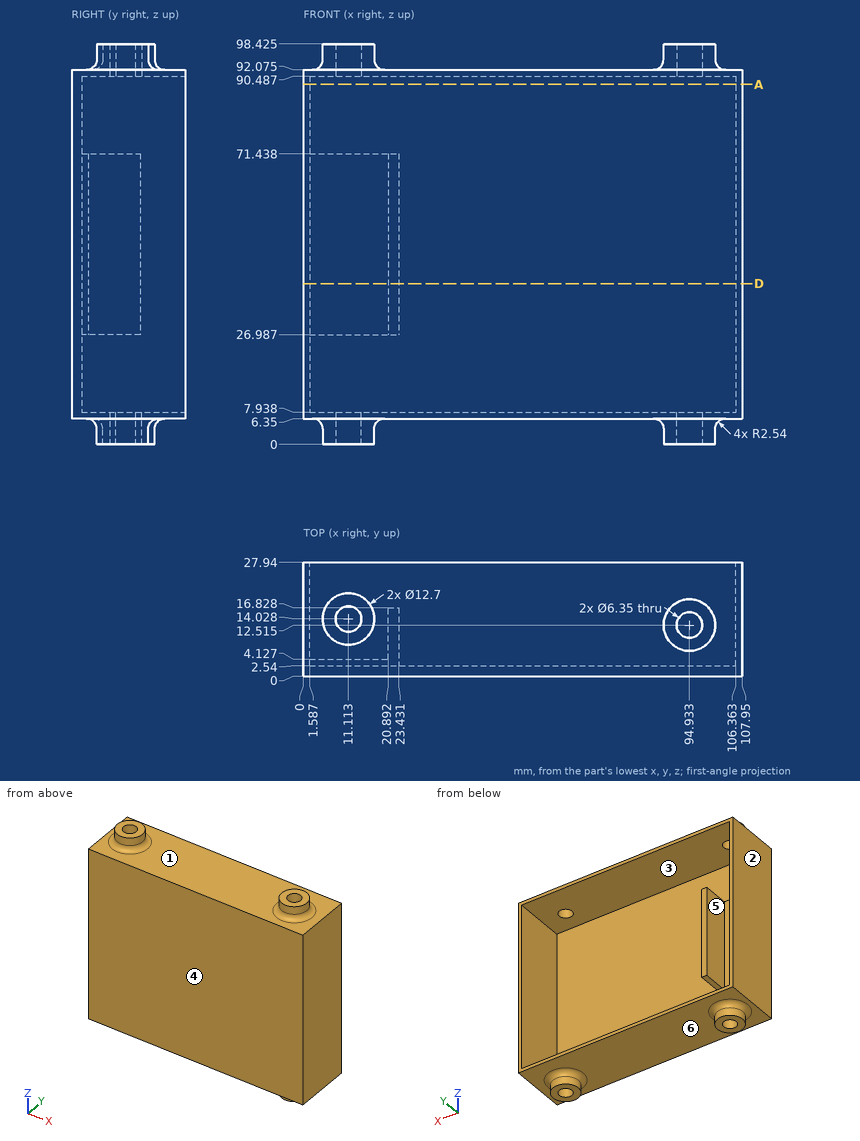
Source: three-view drawing plus pictorial views. Frame: mm from the lowest corner of the part. A direction names the side the tool comes from. Round coordinates to 2 decimals unless told otherwise and drop trailing zeros. Loops run counter-clockwise (first coordinate to the right, second up) from the corner with the lowest first, then second, coordinate; pieces in that order, holes last.
1. Access query for the marked faces 1, 2 and 3. Directions: +Z, -Z, +X, -X, +Y, -Y. A direction counts if a zero-diameter tool reaches every point of the face in a straight line with its end or side. Return the directions, or none.
2. Section query D-D on z = 39.5. Output: boundary loops of the cut face in (x, y).
3. Contact query for flat-ended pins moving along their axis: pin 1 (5.5 mm diameter, centred on x = 11.11, y = 14.03, fed in from +Z) (3 decimals); pin 2 (4 mm diameter, centred on y = 10, z = 51.5, fed in from -X); pin 3 (12.5 mm diameter, centred on x = 54.5, y = 20.5, fed in from -Z); pin 4 (12 mm diameter, centred on x = 40.5, z = 73, fed in from +Y). Output: stop coordinate, or through.
4. Section query A-A on z = 88.5. Output: boundary loops of the cut face in (x, y).
5. Mould query, pull axis Z, two halves, no side actions, for the marked faces 4, 5 and 6. Classes: released by +Z, released by -Z, zero draft, split by the parting line, or undercut.
6. Ray query, L1, parallel to X at y = 11.25, z = 49; L2, parallel to X at y = 12.75, z = 77; L3, parallel to Y at x = 42, z = 45. Return the intervals inside material, ascending.
Answers below:
1. face 1: +Z
1. face 2: +Z, -Z, -X, +Y, -Y
1. face 3: +Y
2. outline: (0, 0) - (107.95, 0) - (107.95, 27.94) - (106.36, 27.94) - (106.36, 2.54) - (23.43, 2.54) - (23.43, 16.83) - (20.89, 16.83) - (20.89, 4.13) - (1.59, 4.13) - (1.59, 27.94) - (0, 27.94) - close
3. pin 1: passes through
3. pin 2: stops at x = 0
3. pin 3: stops at z = 6.35
3. pin 4: stops at y = 2.54
4. outline: (0, 0) - (107.95, 0) - (107.95, 27.94) - (106.36, 27.94) - (106.36, 2.54) - (1.59, 2.54) - (1.59, 27.94) - (0, 27.94) - close
5. face 4: zero draft
5. face 5: undercut
5. face 6: released by -Z
6. L1: x = 0 to 1.59, 20.89 to 23.43, 106.36 to 107.95
6. L2: x = 0 to 1.59, 106.36 to 107.95
6. L3: y = 0 to 2.54
